Build history of the part. All positions in model axes, mm. A direction names the side the tool comes from. Round coordinates to 2 decimals unless told otherwise and drop trailing zeros. Order: outer loops, then holes, each group sorted by start corner. A loop starts at its lowest first (then second) coordinate and runs counter-clockwise, first axis right, second up. Notation, with made-up numbers: (7.5, -36.75) -> (24.5, -36.75) arc R6 cw to (24.5, -29.75) -> close; hole circle Ø3 at (47.5, 86). An arc over 180 degrees is marked (long way). Answer as a JSON object with one key per item and string values.
from build123d import *

# Parameters (mm, degrees)
BOSS_EXTRUDE1_DEPTH                     = 25
FILLET1_R                               = 1
CUT_EXTRUDE2_DEPTH                      = 63.343102097
CBORE_FOR_M5_HEX_HEAD_BOLT1_D           = 5.5
CBORE_FOR_M5_HEX_HEAD_BOLT1_CBORE_D     = 9.5
CBORE_FOR_M5_HEX_HEAD_BOLT1_CBORE_DEPTH = 15
F_5_0_5_DIAMETER_HOLE1_D                = 5
F_5_0_5_DIAMETER_HOLE1_DEPTH            = 15
F_5_0_5_DIAMETER_HOLE1_TIP              = 1.502151548
CHAMFER4_SIZE                           = 1
CHAMFER5_SIZE                           = 1
CHAMFER6_SIZE                           = 1
CHAMFER7_SIZE                           = 1
CHAMFER8_SIZE                           = 1
CHAMFER9_SIZE                           = 1


with BuildPart() as part:
    # Sketch1 → Boss-Extrude1 (new body)
    with BuildSketch(Plane.XY):
        with BuildLine():
            Line((23.483773769, 0.425913311), (8.483773769, 0.425913311))
            Line((8.483773769, 0.425913311), (-7.578534855, -11.620818157))
            ThreePointArc((-7.578534855, -11.620818157), (-11.516226231, -8.324086689), (-15.453917607, -11.620818157))
            Line((-15.453917607, -11.620818157), (-31.516226231, 0.425913311))
            Line((-31.516226231, 0.425913311), (-46.516226231, 0.425913311))
            Line((-46.516226231, 0.425913311), (-46.516226231, 20.425913311))
            Line((-46.516226231, 20.425913311), (-29.849559564, 20.425913311))
            Line((-29.849559564, 20.425913311), (-29.849559564, 5.425913311))
            Line((-29.849559564, 5.425913311), (-16.325743301, -4.716948887))
            ThreePointArc((-16.325743301, -4.716948887), (-11.516226231, -3.324086689), (-6.706709161, -4.716948887))
            Line((-6.706709161, -4.716948887), (6.817107102, 5.425913311))
            Line((6.817107102, 5.425913311), (23.483773769, 5.425913311))
            Line((23.483773769, 5.425913311), (23.483773769, 0.425913311))
        make_face()
    extrude(amount=BOSS_EXTRUDE1_DEPTH)

    # Fillet1
    fillet1_edges = [part.edges().sort_by_distance(p)[0] for p in [
        (-7.578534855, -11.620818157, 12.5),
        (-15.453917607, -11.620818157, 12.5),
    ]]
    fillet(fillet1_edges, radius=FILLET1_R)

    # Sketch5 → Cut-Extrude2 (cut, through all)
    with BuildSketch(Plane(origin=(-29.849559564, 0, 0), x_dir=(0, 0, -1), z_dir=(1, 0, 0))):
        Polygon((0, 7.925913311), (0, 17.925913311), (-1.586948369, 12.925913311), align=None)
        Polygon((-25, 7.925913311), (-25, 17.925913311), (-23.413051631, 12.925913311), align=None)
    extrude(amount=-CUT_EXTRUDE2_DEPTH, mode=Mode.SUBTRACT)

    # CBORE for M5 Hex Head Bolt1 (through all)
    with Locations(Plane(origin=(0, 20.425913311, 0), x_dir=(1, 0, 0), z_dir=(0, 1, 0))):
        with Locations((-40.016226231, -12.5)):
            CounterBoreHole(CBORE_FOR_M5_HEX_HEAD_BOLT1_D / 2, CBORE_FOR_M5_HEX_HEAD_BOLT1_CBORE_D / 2, CBORE_FOR_M5_HEX_HEAD_BOLT1_CBORE_DEPTH)

    # Ø5.0 (5) Diameter Hole1
    with Locations(Plane(origin=(0, 5.425913311, 0), x_dir=(1, 0, 0), z_dir=(0, 1, 0))):
        with Locations((17.483773769, -12.5)):
            Hole(F_5_0_5_DIAMETER_HOLE1_D / 2, depth=F_5_0_5_DIAMETER_HOLE1_DEPTH)
            with Locations((0, 0, -(F_5_0_5_DIAMETER_HOLE1_DEPTH + F_5_0_5_DIAMETER_HOLE1_TIP / 2))):  # 118° drill point
                Cone(0, F_5_0_5_DIAMETER_HOLE1_D / 2, F_5_0_5_DIAMETER_HOLE1_TIP, mode=Mode.SUBTRACT)

    # Chamfer4
    chamfer4_edges = [part.edges().sort_by_distance(p)[0] for p in [
        (-46.516226231, 20.425913311, 12.5),
        (-29.849559564, 20.425913311, 12.5),
    ]]
    chamfer(chamfer4_edges, length=CHAMFER4_SIZE)

    # Chamfer5
    chamfer5_edges = [part.edges().sort_by_distance(p)[0] for p in [
        (-38.182892898, 20.425913311, 25),
        (-38.182892898, 20.425913311, 0),
    ]]
    chamfer(chamfer5_edges, length=CHAMFER5_SIZE)

    # Chamfer6
    chamfer6_edges = [part.edges().sort_by_distance(p)[0] for p in [
        (-46.516226231, 4.175913311, 0),
        (-46.516226231, 15.425913311, 0.793474184),
        (-46.516226231, 10.425913311, 0.793474184),
        (-46.516226231, 18.675913311, 0),
    ]]
    chamfer(chamfer6_edges, length=CHAMFER6_SIZE)

    # Chamfer7
    chamfer7_edges = [part.edges().sort_by_distance(p)[0] for p in [
        (-46.516226231, 4.175913311, 25),
        (-46.516226231, 10.425913311, 24.206525816),
        (-46.516226231, 15.425913311, 24.206525816),
        (-46.516226231, 18.675913311, 25),
    ]]
    chamfer(chamfer7_edges, length=CHAMFER7_SIZE)

    # Chamfer8
    chamfer8_edges = [part.edges().sort_by_distance(p)[0] for p in [
        (-29.849559564, 6.675913311, 0),
        (-29.849559564, 6.675913311, 25),
        (-29.849559564, 18.675913311, 0),
        (-29.849559564, 18.675913311, 25),
        (-29.849559564, 15.425913311, 0.793474184),
        (-29.849559564, 10.425913311, 0.793474184),
        (-29.849559564, 10.425913311, 24.206525816),
        (-29.849559564, 15.425913311, 24.206525816),
    ]]
    chamfer(chamfer8_edges, length=CHAMFER8_SIZE)

    # Chamfer9
    chamfer9_edges = [part.edges().sort_by_distance(p)[0] for p in [
        (15.150440436, 5.425913311, 0),
        (23.483773769, 5.425913311, 12.5),
        (15.150440436, 5.425913311, 25),
    ]]
    chamfer(chamfer9_edges, length=CHAMFER9_SIZE)


solid = part.part
1) Which spindle directions (+Z, -Z, +X, -X, +Y, -Y) get a long thin tool onto all of the face, cutting with end or side? Do faces 4 (the face through (-30.34, 10.46, 23.66)), 5 (the face through (-46.01, 15.39, 1.32)), 6 (the face through (-30.343, 15.465, 1.313)), 7 (the face through (-37, 0.426, 12)). Say none if no direction does.
Checked values:
{"face 4": "+Z, +X", "face 5": "-Z, -X", "face 6": "-Z, +X", "face 7": "+Z, -Z, -X, -Y"}
2) Cut at C-C, the plane z = 20. Give the cut face in (x, y).
Checked values:
{"outline": "(-46.52, 0.43) -> (-31.52, 0.43) -> (-16.54, -10.8) arc R1 ccw to (-15.06, -10.47) arc R4 cw to (-7.97, -10.47) arc R1 ccw to (-6.49, -10.8) -> (8.48, 0.43) -> (23.48, 0.43) -> (23.48, 4.43) -> (22.48, 5.43) -> (6.82, 5.43) -> (-6.71, -4.72) arc R9 ccw to (-16.33, -4.72) -> (-29.85, 5.43) -> (-29.85, 19.43) -> (-30.85, 20.43) -> (-45.52, 20.43) -> (-46.52, 19.43) -> close"}
3) Probe L1, parallel to Y at x = -34.5, z = 2.25; L2, parallel to Z at x = -38.5, y = 19; L3, parallel to Y at x = 12, z = 3. List the from-to ranges inside material, lowest first. Write a range as from..to.
Checked values:
{"L1": "y = 0.43..20.43", "L2": "z = 0..8, 17..25", "L3": "y = 0.43..5.43"}
4) Cut at A-A, the plane z = 12.5. Count the separate pieces of the cut face and the enclosed holes in it, plus the area to 3 significant figures.
Checked values:
{"separate pieces": "3", "enclosed holes": "0", "area": "446 mm²"}
5) Flat gauge pins, fed straight in: pin 1 Ø2 at (x, y) = (-38, 10.5) entering from +Z; pin 2 Ø4 at (x, y) = (-29.5, 11.5) entering from -Z; pin 3 Ø4 at (y, z) = (14, 13) entering from +X; pin 4 Ø5 at (x, z) = (-41.5, 14.5) entering from +Y. Where does each tip first touch, or does it go through?
Checked values:
{"pin 1": "stops at z = 24.5", "pin 2": "stops at z = 0.67", "pin 3": "stops at x = -29.85", "pin 4": "stops at y = 20.43"}
6) Cut at B-B, the plane y = 16. Give the cut face in (x, z).
Checked values:
{"outline": "(-46.52, 1.66) -> (-45.52, 0.61) -> (-30.85, 0.61) -> (-29.85, 1.66) -> (-29.85, 23.34) -> (-30.85, 24.39) -> (-45.52, 24.39) -> (-46.52, 23.34) -> close; hole circle Ø9.5 at (-40.02, 12.5)"}
7) Pull direction Z, two halves, no side cores. Call faces 1 (the face through (-46.01, 15.39, 23.68)), 2 (the face through (-38, 5.426, 15)), 3 (the face through (23.484, 2, 12)): pulls with the +Z half, pulls with the -Z half, needs draft (parallel to the pull), parting line crosses it, or undercut.
Checked values:
{"face 1": "pulls with the +Z half", "face 2": "undercut", "face 3": "needs draft"}
